```python
from build123d import *

# Parameters (mm, degrees)
SKETCH1_W           = 60
SKETCH1_H           = 42
SKETCH1_R           = 12.5
SKETCH1_R_2         = 3
BOSS_EXTRUDE1_DEPTH = 4
FILLET2_R           = 3


with BuildPart() as part:
    # Sketch1 → Boss-Extrude1 (new body)
    with BuildSketch(Plane(origin=(0, 0, 0), x_dir=(1, 0, 0), z_dir=(0, 1, 0))):
        Rectangle(SKETCH1_W, SKETCH1_H)
        with Locations((9, 0)):
            Circle(SKETCH1_R, mode=Mode.SUBTRACT)
        with Locations((-22, 12.25)):
            Circle(SKETCH1_R_2, mode=Mode.SUBTRACT)
        with Locations((-22, -12.25)):
            Circle(SKETCH1_R_2, mode=Mode.SUBTRACT)
    extrude(amount=BOSS_EXTRUDE1_DEPTH)

    # Fillet2
    fillet2_edges = [part.edges().sort_by_distance(p)[0] for p in [
        (30, 2, 21),
        (-30, 2, 21),
        (-30, 2, -21),
        (30, 2, -21),
    ]]
    fillet(fillet2_edges, radius=FILLET2_R)


solid = part.part
```
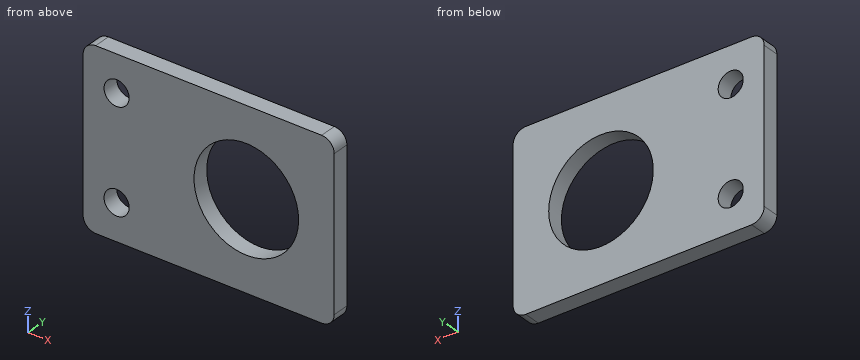
Read the model definition and answer for the solid it produces. Units are mm, in the model's axes. Give positions to 0.01 mm unless a question says otherwise; leave off trailing zeros. Write each loop counter-clockwise with the first axis right and the second up, starting at its lowest first coordinate (ties: lowest second). Pieces come first, ordered by that corner, then holes. Notation, with made-up numbers: (58, -15) -> (67, -15) arc R12 cw to (67, -4) -> close; hole circle Ø11 at (-19.75, -37.5). An arc over 180 degrees is marked (long way). Answer as a JSON object with one key per item and string values.
1) Section C-C on x = -22 is taken. Write down the section's boundary in (y, z).
Findings below:
{"outline": "(0, -21) -> (4, -21) -> (4, -15.25) -> (0, -15.25) -> close; (0, -9.25) -> (4, -9.25) -> (4, 9.25) -> (0, 9.25) -> close; (0, 15.25) -> (4, 15.25) -> (4, 21) -> (0, 21) -> close"}
2) Straight lines are drawn through the part: probe 1 along Z at (x, y) = (-22, 2.35); probe 2 along Z at (x, y) = (9, 2.65); probe 3 along X at (y, z) = (2.5, 0). For each, find the intervals that lie inside material, in ascending order. Write a range as from..to.
Findings below:
{"probe 1": "z = -21..-15.25, -9.25..9.25, 15.25..21", "probe 2": "z = -21..-12.5, 12.5..21", "probe 3": "x = -30..-3.5, 21.5..30"}
3) Section A-A on x = 9 is taken. Write down the section's boundary in (y, z).
Findings below:
{"outline": "(0, -21) -> (4, -21) -> (4, -12.5) -> (0, -12.5) -> close; (0, 12.5) -> (4, 12.5) -> (4, 21) -> (0, 21) -> close"}
4) Section B-B on z = 0 is taken. Write down the section's boundary in (x, y).
Findings below:
{"outline": "(-30, 0) -> (-3.5, 0) -> (-3.5, 4) -> (-30, 4) -> close; (21.5, 0) -> (30, 0) -> (30, 4) -> (21.5, 4) -> close"}
5) Section D-D on z = 10 is taken. Write down the section's boundary in (x, y), then the cut area to 3 significant figures.
Findings below:
{"outline": "(-30, 0) -> (-23.98, 0) -> (-23.98, 4) -> (-30, 4) -> close; (-20.02, 0) -> (1.5, 0) -> (1.5, 4) -> (-20.02, 4) -> close; (16.5, 0) -> (30, 0) -> (30, 4) -> (16.5, 4) -> close", "area": "164 mm^2"}
